from build123d import *

# Parameters (mm, degrees)
SKETCH1_R           = 2.2
SKETCH1_R_2         = 12
BOSS_EXTRUDE1_DEPTH = 7
SKETCH2_W           = 48
SKETCH2_H           = 6
BOSS_EXTRUDE2_DEPTH = 80
BOSS_EXTRUDE3_DEPTH = 48
SKETCH5_W           = 40
SKETCH5_H           = 8
CUT_EXTRUDE1_DEPTH  = 80
SKETCH6_R           = 2.5
CUT_EXTRUDE2_DEPTH  = 80
FILLET1_R           = 5
FILLET5_R           = 4


with BuildPart() as part:
    # Sketch1 → Boss-Extrude1 (new body)
    with BuildSketch(Plane(origin=(0, 0, 0), x_dir=(1, 0, 0), z_dir=(0, 1, 0))):
        with BuildLine():
            Line((5, 0), (63, 0))
            ThreePointArc((63, 0), (66.535533906, 1.464466094), (68, 5))
            Line((68, 5), (68, 63))
            ThreePointArc((68, 63), (66.535533906, 66.535533906), (63, 68))
            Line((63, 68), (5, 68))
            ThreePointArc((5, 68), (1.464466094, 66.535533906), (0, 63))
            Line((0, 63), (0, 5))
            ThreePointArc((0, 5), (1.464466094, 1.464466094), (5, 0))
        make_face()
        with Locations(Location((6, 6, 0), (0, 0, 270))):
            Circle(SKETCH1_R, mode=Mode.SUBTRACT)
        with Locations(Location((62, 6, 0), (0, 0, 270))):
            Circle(SKETCH1_R, mode=Mode.SUBTRACT)
        with Locations(Location((62, 34, 0), (0, 0, 270))):
            Circle(SKETCH1_R, mode=Mode.SUBTRACT)
        with Locations(Location((62, 62, 0), (0, 0, 270))):
            Circle(SKETCH1_R, mode=Mode.SUBTRACT)
        with Locations(Location((6, 34, 0), (0, 0, 270))):
            Circle(SKETCH1_R, mode=Mode.SUBTRACT)
        with Locations(Location((6, 62, 0), (0, 0, 270))):
            Circle(SKETCH1_R, mode=Mode.SUBTRACT)
        with Locations(Location((34, 34, 0), (0, 0, 270))):
            Circle(SKETCH1_R_2, mode=Mode.SUBTRACT)
    extrude(amount=BOSS_EXTRUDE1_DEPTH)

    # Sketch2 → Boss-Extrude2 (add)
    with BuildSketch(Plane(origin=(0, 7, 0), x_dir=(1, 0, 0), z_dir=(0, 1, 0))):
        with Locations((34, 57)):
            Rectangle(SKETCH2_W, SKETCH2_H)
        with Locations((34, 11)):
            Rectangle(SKETCH2_W, SKETCH2_H)
    extrude(amount=BOSS_EXTRUDE2_DEPTH)

    # Sketch4 → Boss-Extrude3 (add)
    with BuildSketch(Plane(origin=(58, 0, 0), x_dir=(0, 0, -1), z_dir=(1, 0, 0))):
        Polygon((8, 7), (0, 7), (8, 87), align=None)
        Polygon((60, 7), (60, 87), (68, 7), align=None)
    extrude(amount=-BOSS_EXTRUDE3_DEPTH)

    # Sketch5 → Cut-Extrude1 (cut)
    with BuildSketch(Plane(origin=(0, 87, 0), x_dir=(1, 0, 0), z_dir=(0, 1, 0))):
        with Locations((34, 64)):
            Rectangle(SKETCH5_W, SKETCH5_H)
        with Locations((34, 4)):
            Rectangle(SKETCH5_W, SKETCH5_H)
    extrude(amount=-CUT_EXTRUDE1_DEPTH, mode=Mode.SUBTRACT)

    # Sketch6 → Cut-Extrude2 (cut)
    with BuildSketch(Plane.XY.offset(-8)):
        with Locations((19, 79)):
            Circle(SKETCH6_R)
        with Locations((49, 79)):
            Circle(SKETCH6_R)
        with Locations((19, 27)):
            Circle(SKETCH6_R)
        with Locations((49, 27)):
            Circle(SKETCH6_R)
    extrude(amount=-CUT_EXTRUDE2_DEPTH, mode=Mode.SUBTRACT)

    # Fillet1
    fillet1_edges = [part.edges().sort_by_distance(p)[0] for p in [
        (34, 7, -54),
        (34, 7, -14),
    ]]
    fillet(fillet1_edges, radius=FILLET1_R)

    # Fillet5
    fillet5_edges = [part.edges().sort_by_distance(p)[0] for p in [
        (14, 7, -64),
        (54, 7, -64),
        (34, 7, -60),
        (14, 7, -4),
        (34, 7, -8),
        (54, 7, -4),
    ]]
    fillet(fillet5_edges, radius=FILLET5_R)


solid = part.part
Geometry check sheet. Reference: the model listing, model coordinates, mm. A direction names the side the tool comes from. Round coordinates to 2 decimals unless told otherwise and drop trailing zeros. Order: outer loops, then holes, each group sorted by start corner. A loop starts at its lowest first (then second) coordinate and runs counter-clockwise, first axis right, second up. Notation, with made-up numbers: M 24.5,26 L 36.5,26 A9 cw 36.5,31 Z; hole C 29,70.25 d2. An arc over 180 degrees is marked long. Answer in a Markdown table with one row per item. Add a question column.
Item 1: Set-up check for faces 4 (the face through (34.28, 8.203, -61.141)), 5 (the face through (34, 7, -2)), 6 (the face through (34, 8, -52)), 7 (the face through (58, 39, -10)): record each of +Z, -Z, +X, -X, +Y, -Y from which the full face is reachable in a straight line by a thin tool's end or side.
Item 2: Depth check by flat-ended pin: pin 1 Ø4 at (y, z) = (40, -4.5) entering from -X; pin 2 Ø3.5 at (x, z) = (6, -34) entering from -Y; pin 3 Ø6 at (x, y) = (43, 23.5) entering from -Z; pin 4 Ø6 at (x, y) = (52, 66.5) entering from +Z. Enter the tip coordinate at first touch or a pass-through.
Item 3: Sectioned sample at C-C, the plane y = 32. Enter the section's corners in (x, z).
Item 4: Sectioned sample at D-D, the plane y = 67. Enter the section's corners in (x, z), plus the area to 3 significant figures.
Item 5: Sectioned sample at B-B, the plane z = -34. Enter the section's corners in (x, y), plus the area to 3 significant figures.
Item 6: Draft check along Y on faces 1 (the face through (33.5, 7, -19.4)), 2 (the face through (34, 3, 0)), 3 (the face through (51.31, 78.04, -10.96)). Enter one of: released by +Y, released by -Y, zero draft, split by the parting line, or undercut.
Item 7: Material ranges on L1, parallel to X at y = 4, z = -6; L2, parallel to X at y = 3.75, z = -34; L3, parallel to Y at x = 49, z = -12.5, recorded low to high. Write a range as [from, to].
Item 8: Sectioned sample at A-A, the plane x = 34. Enter the section's corners in (y, z), plus the area to 3 significant figures.
Filled in:
| question | item | result |
|---|---|---|
| 1 | face 4 | -Z, +Y |
| 1 | face 5 | +Z, +Y |
| 1 | face 6 | +X, -X, +Y |
| 1 | face 7 | +Z, -Z, +X, +Y |
| 2 | pin 1 | stops at x = 10 |
| 2 | pin 2 | passes through |
| 2 | pin 3 | stops at z = -60 |
| 2 | pin 4 | stops at z = -5.73 |
| 3 | outline | M 10,-65.5 L 14,-65.5 L 14,-60 L 54,-60 L 54,-65.5 L 58,-65.5 L 58,-54 L 10,-54 Z; M 10,-14 L 58,-14 L 58,-2.5 L 54,-2.5 L 54,-8 L 14,-8 L 14,-2.5 L 10,-2.5 Z |
| 4 | outline | M 10,-62 L 14,-62 L 14,-60 L 54,-60 L 54,-62 L 58,-62 L 58,-54 L 10,-54 Z; M 10,-14 L 58,-14 L 58,-6 L 54,-6 L 54,-8 L 14,-8 L 14,-6 L 10,-6 Z |
| 4 | area | 608 mm² |
| 5 | outline | M 0,0 L 3.8,0 L 3.8,7 L 0,7 Z; M 8.2,0 L 22,0 L 22,7 L 8.2,7 Z; M 46,0 L 59.8,0 L 59.8,7 L 46,7 Z; M 64.2,0 L 68,0 L 68,7 L 64.2,7 Z |
| 5 | area | 246 mm² |
| 6 | face 1 | released by +Y |
| 6 | face 2 | zero draft |
| 6 | face 3 | undercut |
| 7 | L1 | x = [0, 3.8], [8.2, 59.8], [64.2, 68] |
| 7 | L2 | x = [0, 3.8], [8.2, 22], [46, 59.8], [64.2, 68] |
| 7 | L3 | y = [0, 24.5], [29.5, 76.5], [81.5, 87] |
| 8 | outline | M 0,-68 L 7,-68 L 7,-64 A4 cw 11,-60 L 87,-60 L 87,-54 L 12,-54 A5 cw 7,-49 L 7,-46 L 0,-46 Z; M 0,-22 L 7,-22 L 7,-19 A5 cw 12,-14 L 87,-14 L 87,-8 L 11,-8 A4 cw 7,-4 L 7,0 L 0,0 Z |
| 8 | area | 1,290 mm² |
